Autodesk Inventor part; units mm, degrees
ref_plane "Work Plane2" through (-13.9845, -14.3768, -78) normal (0, 0, -1) x (0, 1, 0)
ref_plane "YZ Plane" through (0, 0, 0) normal (1, 0, 0) x (0, 1, 0)
ref_plane "XZ Plane" through (0, 0, 0) normal (0, 1, 0) x (-1, 0, 0)
ref_plane "Work Plane1" through (-0.1632, 0, 0) normal (0, 0, 1) x (1, 0, 0)
sketch "Sketch1" plane through (-0.1632, 0, 0) normal (0, 0, 1) x (1, 0, 0)
  circle A0 centre (9.6632, 0) radius 1.5
  line L0 (12.6832, 3.5) -> (9.6632, 3.5)
  arc A1 (9.6632, 3.5) -> (9.6632, -3.5) centre (9.6632, 0) ccw
  line L1 (9.6632, -3.5) -> (12.6832, -3.5)
  arc A2 (12.6832, -3.5) -> (12.6832, 3.5) centre (0.1632, 0) ccw
  circle A3 centre (0.1788, -0.3768) radius 14
  circle A4 centre (0.1788, -0.3768) radius 11
  line L2 (12.6832, -3.5) -> (18.2293, -3.5)
  line L3 (12.6832, 3.5) -> (18.7282, 3.5)
  circle A5 centre (0.1788, -0.3768) radius 16.5
  line L4 (16.6788, -0.3768) -> (20.6788, -0.3768)
  circle A6 centre (0.1788, -0.3768) radius 20.5
  line L5 (18.7282, 3.5) -> (20.3088, 3.5)
  line L6 (18.2293, -3.5) -> (20.4394, -3.5)
  point P0 (0.1632, 0)
  dimension "d0" = 33
  dimension "d1" = 4
extrude "Extrusion1" add sketch "Sketch1" along normal blind 3.5 contours A2 L1 A4 L0 | L3 A3 L2 A2 | A4 L1 A1 L0 | L3 A5 L2 A3 | L3 L5 A6 L4 A5 | A5 L4 A6 L6 L2 picked at (10.1281, -2.4909) picked at (14.5943, 3.0756)
sketch "Sketch2" plane through (-0.1632, 0, 0) normal (0, 0, -1) x (-1, 0, 0)
  line L0 (-9.6632, -3.5) -> (-20.4394, -3.5)
  arc A0 (-9.6632, -3.5) -> (-9.6632, 3.5) centre (-9.6632, 0) ccw
  line L1 (-20.3088, 3.5) -> (-9.6632, 3.5)
  arc A1 (-20.3088, 3.5) -> (-20.4394, -3.5) centre (-0.1788, -0.3768) ccw
  circle A2 centre (-9.6632, 0) radius 1.5
  circle A3 centre (-0.1788, -0.3768) radius 14
  line L2 (-14.1788, -0.3768) -> (-16.1788, -0.3768)
  circle A4 centre (-0.1788, -0.3768) radius 16
  line L3 (-16.1788, -0.3768) -> (-19.6788, -0.3768)
  circle A5 centre (-0.1788, -0.3768) radius 19.5
  circle A6 centre (-0.1788, -0.3768) radius 2
  point P0 (-0.1632, 0)
  point P1 (-19.427, -3.5)
  point P2 (-15.871, -3.5)
  point P3 (-15.702, 3.5)
  point P4 (-19.2895, 3.5)
  dimension "d4" = 2
  dimension "d5" = 3.5
ref_plane "Work Plane2" through (-13.9845, -14.3768, -78) normal (0, 0, -1) x (0, 1, 0)
extrude "Extrusion2" add sketch "Sketch2" along normal blind 83.5 contours L0 A5 L3 A4 | L3 A5 L1 A4
sketch "Sketch3" plane through (-0.1632, 0, -83.5) normal (0, 0, -1) x (-1, 0, 0)
  circle A0 centre (-0.1788, -0.3768) radius 14
  circle A1 centre (-9.6632, 0) radius 1.5
  arc A2 (-15.702, 3.5) -> (-15.871, -3.5) centre (-0.1788, -0.3768) ccw
  line L0 (-9.6632, -3.5) -> (-15.871, -3.5)
  arc A3 (-9.6632, -3.5) -> (-9.6632, 3.5) centre (-9.6632, 0) ccw
  line L1 (-15.702, 3.5) -> (-9.6632, 3.5)
  circle A4 centre (-0.1788, -0.3768) radius 2
  arc A5 (-9.6632, -3.5) -> (-9.6632, 3.5) centre (-9.6632, 0) ccw
  line L2 (-9.6632, 3.5) -> (-12.6832, 3.5)
  arc A6 (-12.6832, -3.5) -> (-12.6832, 3.5) centre (-0.1632, 0) ccw
  line L3 (-12.6832, -3.5) -> (-9.6632, -3.5)
  line L4 (3.8368, -5) -> (-4.1632, -5)
  line L5 (3.8368, 5) -> (3.8368, -5)
  line L6 (-4.1632, 5) -> (3.8368, 5)
  line L7 (-4.1632, -5) -> (-4.1632, 5)
  point P0 (-0.1632, 0)
  dimension "d8" = 4
extrude "Extrusion3" add sketch "Sketch3" against normal blind 4 contours L1 A3 L0 A0 | A0 L0 A2 L1 | A6 L0 A3 L1 | L4 L7 L6 L5
sketch "Sketch4" plane through (-0.1632, 0, 3.5) normal (0, 0, 1) x (1, 0, 0)
  arc A0 (19.427, -3.5) -> (19.2895, 3.5) centre (0.1788, -0.3768) ccw
  arc A1 (19.427, -3.5) -> (19.2895, 3.5) centre (0.1788, -0.3768) ccw
  arc A2 (15.871, -3.5) -> (15.702, 3.5) centre (0.1788, -0.3768) ccw
  line L0 (9.6632, -3.5) -> (20.4394, -3.5)
  arc A3 (20.4394, -3.5) -> (20.3088, 3.5) centre (0.1788, -0.3768) ccw
  line L1 (20.3088, 3.5) -> (9.6632, 3.5)
  arc A4 (9.6632, 3.5) -> (9.6632, -3.5) centre (9.6632, 0) ccw
  circle A5 centre (9.6632, 0) radius 1.5
  point P0 (0.1632, 0)
  point P1 (19.2895, 3.5)
  point P2 (19.427, -3.5)
extrude "Extrusion4" cut sketch "Sketch4" against normal blind 4 contours A0 L1 A3 L0
properties material "PC/ABS Plastic"
CAD build for the part. Positions are in the model's coordinates, mm. A direction names the side the tool comes from. Round coordinates to 2 decimals unless told otherwise and drop trailing zeros. Loops run counter-clockwise (first coordinate to the right, second up) from the corner with the lowest first, then second, coordinate; pieces in that order, holes last. Notation, with made-up numbers: (20, 8) - (67, 8) arc R33 cw to (67, 41) - close; hole circle Ø8 at (28, 40.5). An arc over 180 degrees is marked (long way). Return JSON: item names as keys, results as strings. Group by question number.
Q1. Tool access for faces 1 (the face through (19.513, -0.043, -41.166)), 2 (the face through (6, 0, 2)): list every direction of +Z, -Z, +X, -X, +Y, -Y with a clear straight run to the whole face (end or side of a thin tool).
Q2. Flat gauge pins, fed straight in: pin 1 Ø6 at (x, z) = (13, -24.5) entering from -Y; pin 2 Ø10.5 at (x, z) = (14, -52.5) entering from +Y; pin 3 Ø2 at (x, y) = (8.5, 0.5) entering from -Z; pin 4 Ø3 at (y, z) = (0, -42) entering from -X. Where does each tip first touch, or does it go through?
Q3. Band-saw the part on B-B on y = -8.5. Give the cut face in (x, z).
Q4. Drill centre lines: line 1 along Y through (x, z) = (9.5, 1.95); line 2 along Z through (x, y) = (12.5, 1.25); line 3 along Z through (x, y) = (-2.5, -3). Where is each one in solid material? Low to high. Write a range as [from, to].
Q5. Two-plate mould, pull along Y, no slides. Class faces 3 (the face through (11, 0, -82)), 4 (the face through (17, 3.5, -40)), 5 (the face through (16.012, -0.04, -39.194)), 6 (the face through (-12.99, -0.52, -81.53)): +Y half, -Y half, draft (parallel to the pull), parting line (faces both ways), or undercut.
Q6. Band-saw the part on C-C on z = -56.5. Give the cut face in (x, y).
Q7. Band-saw the part on A-A on x = 0. Give the cut face in (y, z).
Solutions:
{
 "1": {"face 1": "+Z, -Z, +X", "face 2": "+Z, -X"},
 "2": {"pin 1": "stops at y = -3.5", "pin 2": "stops at y = 3.5", "pin 3": "stops at z = -83.5", "pin 4": "stops at x = 15.91"},
 "3": {"outline": "(-9.84, -83.5) - (9.84, -83.5) - (9.84, -79.5) - (-9.84, -79.5) - close"},
 "4": {"line 1": "y = [-3.5, -1.5], [1.5, 3.5]", "line 2": "z = [-83.5, -79.5], [0, 3.5]", "line 3": "z = [-83.5, -79.5]"},
 "5": {"face 3": "undercut", "face 4": "+Y half", "face 5": "undercut", "face 6": "parting line"},
 "6": {"outline": "(15.54, 3.5) arc R16 cw to (15.71, -3.5) - (19.26, -3.5) arc R19.5 ccw to (19.13, 3.5) - close"},
 "7": {"outline": "(-13, -83.5) - (-2.38, -83.5) - (-2.38, -79.5) - (-13, -79.5) - close; (1.62, -83.5) - (13, -83.5) - (13, -79.5) - (1.62, -79.5) - close"}
}
